Could you check a few things on this model? Use its own coordinates, in mm. Face numbers are marked on the shaded views. A direction names the side the tool comes from. Round coordinates to 2 decimals unless told otherwise and drop trailing zeros. Loops run counter-clockwise (first coordinate to the right, second up) from the corner with the lowest first, then second, coordinate; pieces in that order, holes last. Notation, with made-up numbers: M -28.75,-23 L 3.25,-23 A19 ccw 3.25,-10 Z; hole C -10.5,41.25 d4. An arc over 180 degrees is marked long. Return JSON: item names as keys, results as strings. Group by question number.
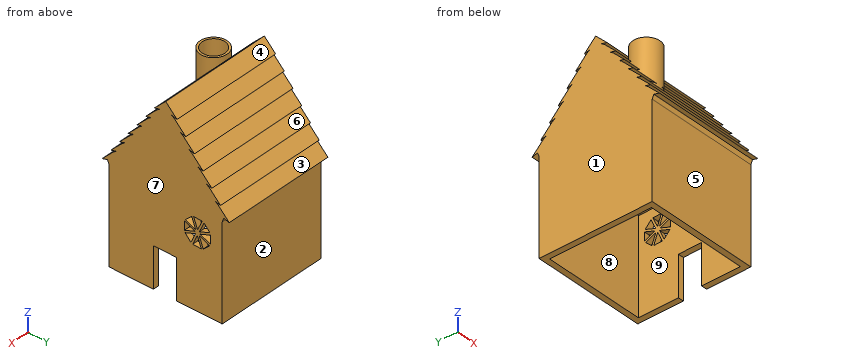
```python
from build123d import *

# Parameters (mm, degrees)
F0_W     = 50.8
F0_H     = 50.8
F0_W_2   = 45.72
F0_H_2   = 45.72
F1_DEPTH = 42.418
F2_W     = 10.449068
F2_H     = 18.06196
F3_DEPTH = 33.02
F5_DEPTH = 50.8
F6_R     = 6.04507
F6_R_2   = 5.111914
F7_DEPTH = 35.56
F9_DEPTH = 25.4


with BuildPart() as f1:
    # F0 (on Top) → F1 (new body)
    with BuildSketch(Plane.XY):
        Rectangle(F0_W, F0_H)
        Rectangle(F0_W_2, F0_H_2, mode=Mode.SUBTRACT)
    extrude(amount=F1_DEPTH)

    # F2 (on face) → F3 (cut)
    with BuildSketch(Plane.YZ.offset(25.4)):
        with Locations((-0.298544, 9.03098)):
            Rectangle(F2_W, F2_H)
    extrude(amount=-F3_DEPTH, mode=Mode.SUBTRACT)

    # F4 (on face) → F5 (join)
    with BuildSketch(Plane.YZ.offset(25.4)):
        Polygon((5.08, 75.438), (0, 80.518), (-5.08, 75.438), (-2.626548, 76.0954), (-3.912723, 75.197905), (-8.992723, 70.117905), (-6.539271, 70.775305), (-7.825446, 69.877809), (-12.905446, 64.797809), (-10.451994, 65.455209), (-11.738169, 64.557714), (-16.818169, 59.477714), (-14.364717, 60.135114), (-15.650891, 59.237618), (-20.730891, 54.157618), (-18.27744, 54.815018), (-19.563614, 53.917523), (-24.643614, 48.837523), (-22.190163, 49.494923), (-23.476337, 48.597427), (-28.556337, 43.517427), (-26.102885, 44.174827), (-25.4, 42.418), (25.4, 42.418), (26.102885, 44.174827), (28.556337, 43.517427), (23.476337, 48.597427), (22.190163, 49.494923), (24.643614, 48.837523), (19.563614, 53.917523), (18.27744, 54.815018), (20.730891, 54.157618), (15.650891, 59.237618), (14.364717, 60.135114), (16.818169, 59.477714), (11.738169, 64.557714), (10.451994, 65.455209), (12.905446, 64.797809), (7.825446, 69.877809), (6.539271, 70.775305), (8.992723, 70.117905), (3.912723, 75.197905), (2.626548, 76.0954), align=None)
    extrude(amount=-F5_DEPTH)

    # F6 (on face) → F7 (join)
    with BuildSketch(Plane(origin=(0, 0, 42.418), x_dir=(1, 0, 0), z_dir=(0, 0, -1))):
        with Locations((-11.792519, 10.896885)):
            Circle(F6_R)
        with Locations((-11.792519, 10.896885)):
            Circle(F6_R_2, mode=Mode.SUBTRACT)
    extrude(amount=-F7_DEPTH)

    # F8 (on face) → F9 (cut)
    with BuildSketch(Plane.YZ.offset(25.4)):
        Polygon((13.460486, 33.579258), (11.696823, 38.290104), (8.882317, 35.663231), align=None)
        Polygon((14.316839, 33.899863), (16.400811, 38.478032), (12.553176, 38.610708), align=None)
        Polygon((15.149074, 33.521031), (19.859919, 35.284695), (17.233046, 38.0992), align=None)
        Polygon((13.081654, 32.747024), (8.503485, 34.830996), (8.370809, 30.98336), align=None)
        Polygon((13.402259, 31.89067), (8.691413, 30.127007), (11.318286, 27.312501), align=None)
        Polygon((14.234494, 31.511839), (12.150521, 26.93367), (15.998157, 26.800994), align=None)
        Polygon((15.090847, 31.832444), (16.85451, 27.121598), (19.669016, 29.748471), align=None)
        Polygon((15.469678, 32.664678), (20.047847, 30.580706), (20.180524, 34.428342), align=None)
    extrude(amount=-F9_DEPTH, mode=Mode.SUBTRACT)


solid = f1.part
```
1. I need wall thicknesses on probe 1 along Y at (x, z) = (-20, 27.5); probe 2 along Y at (x, z) = (23.5, 4). Which ranges of each line are inside material? Lowest first, please.
2. On a 3-axis mill with a long thin cutter (end or side, diameter ignored), from which of +Z, -Z, +X, -X, +Y, -Y can I reach the whole of each face in a straight line? I mean the marked faces 1, 2, 3, 4 and 5. Say none if no direction works.
3. We'd pull the mould along Y, two halves only. Please class the marked faces 6, 7, 8 and 9: +Y half, -Y half, draft (parallel to the pull), parting line (faces both ways), or undercut.
4. I'm going to push flat-ended pins straight in: pin 1 Ø6 at (x, z) = (-13, 70) entering from +Y; pin 2 Ø8 at (x, y) = (-11.79, -10.9) entering from +Z; pin 3 Ø21 at (x, z) = (-8.5, 16) entering from -Y. Where does each tip first touch, or does it pass through?
5. If we section it at A-A, the plane z = 52.5: Please give me the cut outline in (x, y), then the cut area to 3 significant figures.
Geometry results:
{
 "1": {"probe 1": "-25.4 to -22.86, 22.86 to 25.4", "probe 2": "-25.4 to -5.52, 4.93 to 25.4"},
 "2": {"face 1": "+Z, -Z, -X, +Y, -Y", "face 2": "-Z, +X, -X, +Y", "face 3": "+X, -X, +Y", "face 4": "+Z, +X, -X, +Y", "face 5": "-Z, +X, -X, -Y"},
 "3": {"face 6": "+Y half", "face 7": "draft", "face 8": "undercut", "face 9": "undercut"},
 "4": {"pin 1": "y = 10.7", "pin 2": "z = 72.21", "pin 3": "y = -25.4"},
 "5": {"outline": "M -25.4,-20.98 L 25.4,-20.98 L 25.4,20.98 L -25.4,20.98 Z", "area": "2,130 mm^2"}
}
